The drawing under review shows one solid part. Ordinate dimensions are in mm from its lowest x, y, z. Give positions to 0.01 mm unless a question says otherwise; leave off trailing zeros. Loops run counter-clockwise (first coordinate to the right, second up) from the corner with the lowest first, then second, coordinate; pieces in that order, holes last. Notation, with made-up numbers: (-5.5, -26) - (26.5, -26) arc R13 cw to (26.5, -17) - close; hole circle Ø7 at (43.25, 42.5). An arc over 180 degrees is marked (long way). Return JSON: item names as keys, results as strings. Group by question number.
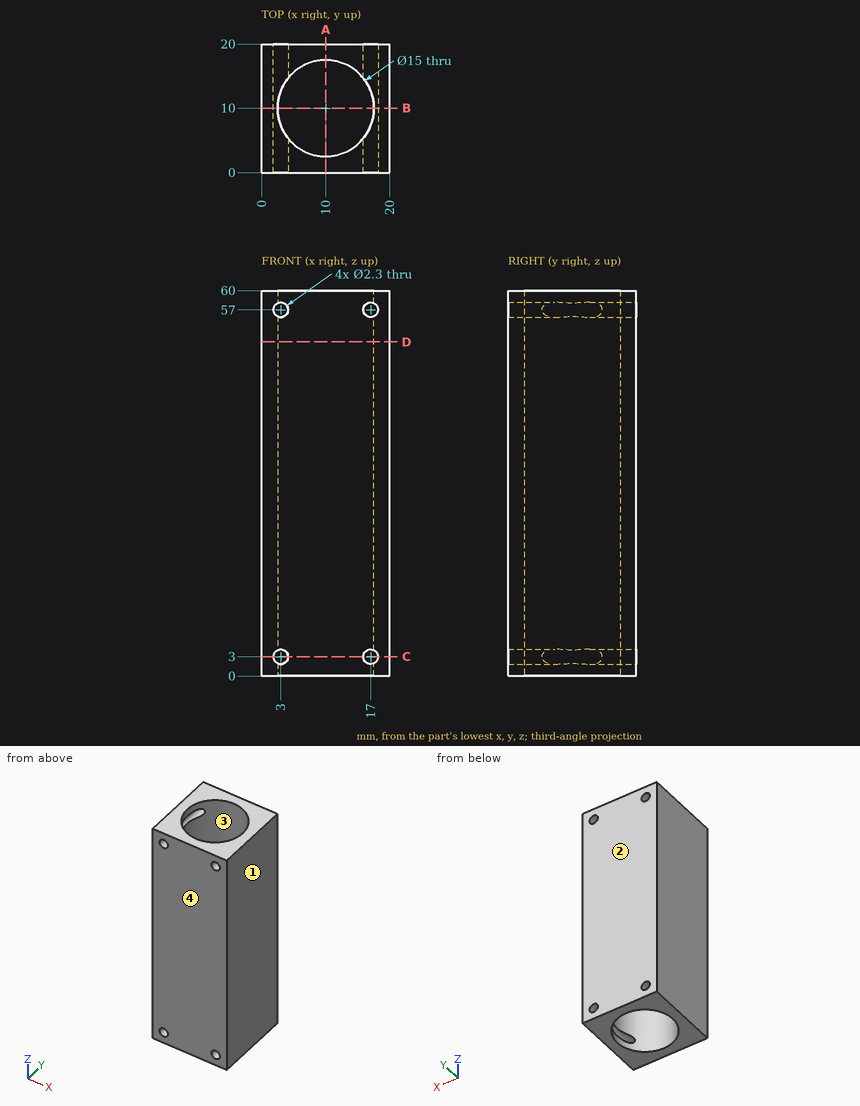
1) We need section A-A, the plane x = 10. Write out the cut boundary in (y, z), plus the area to 3 significant figures.
2) We need section B-B, the plane y = 10. Write out the cut boundary in (x, z), plus the area to 3 significant figures.
3) For pin 1 Ø1.4 at (x, z) = (17, 57) entering from -Y, flat-tipped, find the tip position at first contact; note if it passes through.
4) We need section D-D, the plane z = 52. Write out the cut boundary in (x, y), plus the area to 3 significant figures.
5) Draft analysis for pull direction Y (two halves, no side actions). For the marked faces 1, 2, 3 and 4, state which applies: +Y half, -Y half, draft (parallel to the pull), parting line (faces both ways), or undercut.
6) To check wall thickness, follow line 1 (Z direction, x = 17, y = 6); line 2 (Y direction, x = 10.75, z = 15); line 3 (Z direction, x = 3.5, y = 5.25). State the ranges of each line that lie inside material, in increasing order.
7) We need section C-C, the plane z = 3. Write out the cut boundary in (x, y), plus the area to 3 significant figures.
Findings:
{
 "1": {"outline": "(0, 0) - (2.5, 0) - (2.5, 60) - (0, 60) - close; (17.5, 0) - (20, 0) - (20, 60) - (17.5, 60) - close", "area": "300 mm^2"},
 "2": {"outline": "(0, 0) - (2.5, 0) - (2.5, 1.96) arc R1.15 cw to (2.5, 4.04) - (2.5, 55.96) arc R1.15 cw to (2.5, 58.04) - (2.5, 60) - (0, 60) - close; (17.5, 0) - (20, 0) - (20, 60) - (17.5, 60) - (17.5, 58.04) arc R1.15 cw to (17.5, 55.96) - (17.5, 4.04) arc R1.15 cw to (17.5, 1.96) - close", "area": "296 mm^2"},
 "3": {"pin 1": "passes through"},
 "4": {"outline": "(0, 0) - (20, 0) - (20, 20) - (0, 20) - close; hole circle Ø15 at (10, 10)", "area": "223 mm^2"},
 "5": {"face 1": "draft", "face 2": "+Y half", "face 3": "undercut", "face 4": "-Y half"},
 "6": {"line 1": "z = 0 to 1.85, 4.15 to 55.85, 58.15 to 60", "line 2": "y = 0 to 2.54, 17.46 to 20", "line 3": "z = 0 to 1.96, 4.04 to 55.96, 58.04 to 60"},
 "7": {"outline": "(0, 0) - (1.85, 0) - (1.85, 20) - (0, 20) - close; (4.15, 0) - (15.85, 0) - (15.85, 5.31) arc R7.5 cw to (4.15, 5.31) - close; (4.15, 14.69) arc R7.5 cw to (15.85, 14.69) - (15.85, 20) - (4.15, 20) - close; (18.15, 0) - (20, 0) - (20, 20) - (18.15, 20) - close", "area": "152 mm^2"}
}
